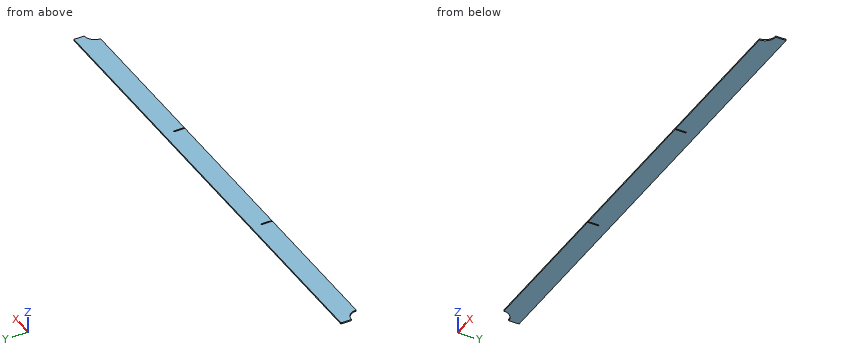
Autodesk Inventor part; units mm, degrees
ref_plane "YZ Plane" through (0, 0, 0) normal (1, 0, 0) x (0, 1, 0)
ref_plane "XZ Plane" through (0, 0, 0) normal (0, 1, 0) x (-1, 0, 0)
ref_plane "XY Plane" through (0, 0, 0) normal (0, 0, 1) x (1, 0, 0)
sketch "Sketch1" plane through (0, 0, 0) normal (0, 0, 1) x (1, 0, 0)
  line L0 (-580, 50) -> (580, 50)
  line L1 (580, 50) -> (580, 0)
  line L2 (580, 0) -> (-580, 0)
  line L3 (-580, 0) -> (-580, 50)
  circle A0 centre (-580, 0) radius 25
  circle A1 centre (580, 0) radius 25
  point P0 (0, 0)
  point P1 (0, 0)
  point P2 (-580, 25)
  point P3 (-555, 0)
  point P4 (555, 0)
  point P5 (580, 25)
  dimension "d16" = 50
  dimension "d17" = 1160
  dimension "d18" = 50
  dimension "d19" = 50
extrude "Plate2" add sketch "Sketch1" against normal blind 3 contours L0 L1 A1 L2 A0 L3
sketch "Sketch2" plane through (0, 0, 0) normal (0, 0, 1) x (1, 0, 0)
  line L0 (-555, 0) -> (555, 0)
  line L1 (190, 0) -> (190, 50) construction
  line L2 (580, 50) -> (-580, 50)
  line L3 (188.5, 26) -> (191.5, 26)
  line L4 (191.5, 26) -> (191.5, 0)
  line L5 (191.5, 0) -> (188.5, 0)
  line L6 (188.5, 0) -> (188.5, 26)
  line L7 (-190, 50) -> (-190, 0) construction
  line L8 (-191.5, 26) -> (-188.5, 26)
  line L9 (-188.5, 26) -> (-188.5, 0)
  line L10 (-188.5, 0) -> (-191.5, 0)
  line L11 (-191.5, 0) -> (-191.5, 26)
  point P0 (0, 0)
  point P1 (0, 0)
  point P2 (191.5, 0)
  point P3 (0, 0)
  point P4 (-188.5, 0)
  dimension "d21" = 190
  dimension "d22" = 3
  dimension "d23" = 26
  dimension "d29" = 190
  dimension "d30" = 3
  dimension "d31" = 26
extrude "Extrusion1" cut sketch "Sketch2" against normal through all
equation "\"d22\" = Thickness"
equation "\"d30\" = Thickness"
equation "\"d31\" = d23"
equation "\"d20\" = Thickness"
equation "\"BendReliefWidth\" = Thickness"
equation "\"BendReliefDepth\" = 0.5 * Thickness"
equation "\"CornerReliefSize\" = 4 * Thickness"
equation "\"MinimumRemnant\" = 2 * Thickness"
equation "\"TransitionRadius\" = BendRadius"
equation "\"JacobiRadiusSize\" = BendRadius"
equation "\"GapSize\" = Thickness"
properties part number "MSC 0563 rib cone" material "Stainless Steel"
Geometry: final body of the model. Coordinates: model frame, mm. Coordinates: 2 decimals unless noted, no trailing zeros. Order: outer loops, then holes, each group sorted by start corner. A loop starts at its lowest first (then second) coordinate and runs counter-clockwise, first axis right, second up.
1) Section A-A (z = -2.1). Return loops of the section in (x, y), then the cut area to 3 significant figures.
Result sheet:
outline: (-580, 25) arc R25 cw to (-555, 0) - (-191.5, 0) - (-191.5, 26) - (-188.5, 26) - (-188.5, 0) - (188.5, 0) - (188.5, 26) - (191.5, 26) - (191.5, 0) - (555, 0) arc R25 cw to (580, 25) - (580, 50) - (-580, 50) - close
area: 56,900 mm2
2) First-contact query: P1, Ø0.9, axis at x = 190.5, z = -1.5, coming from the -Y side; P2, Ø0.9, axis at y = 17, z = -1.5, coming from the +X side; P3, Ø0.9, axis at y = 15.5, z = -1, coming from the -X side. Flat tips, straight axial feed; report the tip coordinate or a pass-through.
Result sheet:
P1: stops at y = 26
P2: stops at x = 562.1
P3: stops at x = -560.75
3) Section B-B (y = 12). Return loops of the section in (x, z).
Result sheet:
outline: (-558.07, -3) - (-191.5, -3) - (-191.5, 0) - (-558.07, 0) - close; (-188.5, -3) - (188.5, -3) - (188.5, 0) - (-188.5, 0) - close; (191.5, -3) - (558.07, -3) - (558.07, 0) - (191.5, 0) - close
4) Ray query, probe 1 along X at (y, z) = (17, -2.05); probe 2 along X at (y, z) = (4, -0.8). Return the intervals inside material, ascending.
Result sheet:
probe 1: x = -561.67 to -191.5, -188.5 to 188.5, 191.5 to 561.67
probe 2: x = -555.32 to -191.5, -188.5 to 188.5, 191.5 to 555.32
